Read the model definition and answer for the solid it produces. Units are mm, in the model's axes. Face numbers are marked on the shaded views. Give positions to 0.01 mm unless a question says otherwise; leave off trailing zeros. Order: outer loops, then holes, each group sorted by start corner. A loop starts at its lowest first (then second) coordinate and runs counter-clockwise, first axis right, second up. Notation, with made-up numbers: (-36, 68) - (13, 68) arc R19 cw to (13, 74) - close; hole circle Ø5 at (65.5, -27.5). An arc over 180 degrees is marked (long way). Return JSON: item names as keys, results as strings.
```python
from build123d import *

# Parameters (mm, degrees)
SKETCH017_R            = 1
PAD017_DEPTH           = 10
CYLINDER032_R          = 2.8
CYLINDER032_DEPTH      = 21
CYLINDER033_R          = 5
CYLINDER033_DEPTH      = 2
CUT015_PITCH_ANGLE     = 90
CUT015_PLACEMENT_ANGLE = -90


with BuildPart() as pad017:
    # Sketch017 → Pad017 (new body)
    with BuildSketch(Plane(origin=(0, 4.2, 21), x_dir=(1, 0, 0), z_dir=(0, -1, 0))):
        Circle(SKETCH017_R)
    extrude(amount=PAD017_DEPTH)


with BuildPart() as eje001:
    # Cylinder032 → Cylinder032 (new body)
    with BuildSketch(Plane.XY.offset(2)):
        Circle(CYLINDER032_R)
    extrude(amount=CYLINDER032_DEPTH)


with BuildPart() as eje_full1:
    # Cylinder033 → Cylinder033 (new body)
    with BuildSketch(Plane.XY):
        Circle(CYLINDER033_R)
    extrude(amount=CYLINDER033_DEPTH)

    # Fusion009003019: union Eje001
    add(eje001.part)

    # Cut015: cut Pad017
    add(pad017.part, mode=Mode.SUBTRACT)


with BuildPart() as eje_full1_1:
    # Cut015 pitch: moved
    add(eje_full1.part.rotate(Axis((0, 0, 0), (0, 1, 0)), CUT015_PITCH_ANGLE))


with BuildPart() as eje_full1_2:
    # Cut015 placement: moved
    add(eje_full1_1.part.moved(Location((367.5, 80, 312))).rotate(Axis((367.5, 80, 312), (0, 0, 1)), CUT015_PLACEMENT_ANGLE))


solid = eje_full1_2.part
```
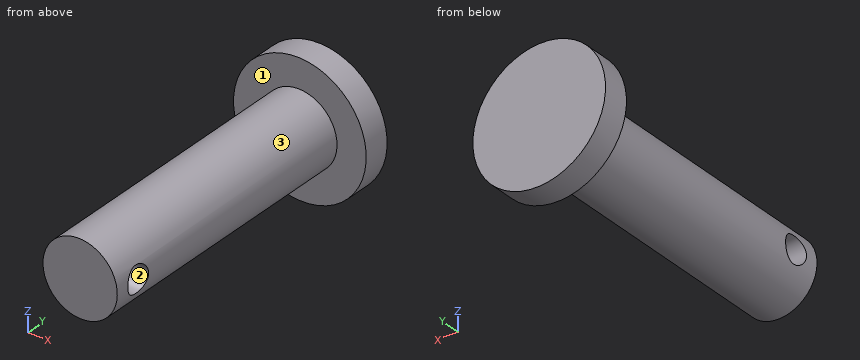
Q1. A cutting plane is placed at C-C (y = 59). Write down the section's boundary in (x, z), and give its area (3 significant figures).
Values:
{"outline": "(364.88, 311) arc R2.8 ccw to (370.12, 311) - close; (364.88, 313) - (370.12, 313) arc R2.8 ccw to start", "area": "13.7 mm²"}
Q2. A cutting plane is placed at A-A (z = 312). Write down the section's boundary in (x, y), and give its area (3 significant figures).
Values:
{"outline": "(362.5, 78) - (364.7, 78) - (364.7, 60) - (370.3, 60) - (370.3, 78) - (372.5, 78) - (372.5, 80) - (362.5, 80) - close; (364.7, 57) - (370.3, 57) - (370.3, 58) - (364.7, 58) - close", "area": "126 mm²"}
Q3. Consider L1, parallel to Y at x = 368.2, z = 312; L2, parallel to Z at x = 367.35, y = 59; L3, parallel to Y at x = 371, z = 309. Determine where each line is inside the solid, lowest interval first.
Values:
{"L1": "y = 57 to 58, 60 to 80", "L2": "z = 309.2 to 311, 313 to 314.8", "L3": "y = 78 to 80"}
Q4. Determine the mould class of the marked faces 1, 2 and 3 for opening direction Z: released by +Z, released by -Z, zero draft, split by the parting line, or undercut.
Values:
{"face 1": "zero draft", "face 2": "undercut", "face 3": "split by the parting line"}
Q5. A cutting plane is placed at D-D (z = 313.5). Write down the section's boundary in (x, y), and give its area (3 significant figures).
Values:
{"outline": "(362.73, 78) - (365.14, 78) - (365.14, 57) - (369.86, 57) - (369.86, 78) - (372.27, 78) - (372.27, 80) - (362.73, 80) - close", "area": "118 mm²"}
Q6. Given pin 1 (1 mm diameter, centred on x = 371, z = 308.5, fed in from -Y); pin 2 (1.5 mm diameter, centred on y = 66, z = 314, fed in from +X); pin 3 (2.5 mm diameter, centred on y = 59, z = 312, fed in from -X), each flat-ended and moving along its own axis, determine where each tip first touches the part or whether it passes through.
Values:
{"pin 1": "stops at y = 78", "pin 2": "stops at x = 370.01", "pin 3": "stops at x = 364.7"}
Q7. A cutting plane is placed at B-B (x = 367.5). Write down the section's boundary in (y, z), and give its area (3 significant figures).
Values:
{"outline": "(57, 309.2) - (78, 309.2) - (78, 307) - (80, 307) - (80, 317) - (78, 317) - (78, 314.8) - (57, 314.8) - close; hole circle Ø2 at (59, 312)", "area": "134 mm²"}
